```python
from build123d import *

# Parameters (mm, degrees)
BOSS_EXTRU_1_DEPTH           = 80
ENL_V_MAT_EXTRU_1_DEPTH      = 95.994736696
D_GAGEMENT_M11_D             = 16
D_GAGEMENT_M11_DEPTH         = 72
D_GAGEMENT_M11_TIP           = 4.618802154
ENL_V_MAT_EXTRU_2_REACH      = 91.582
ENL_V_MAT_EXTRU_2_END_RADIUS = 8
ESQUISSE3_R                  = 5
ENL_V_MAT_EXTRU_3_REACH      = 92.863
ENL_V_MAT_EXTRU_3_END_RADIUS = 8
ESQUISSE7_R                  = 2


with BuildPart() as part:
    # Esquisse1 → Boss.-Extru.1 (new body)
    with BuildSketch(Plane.XY):
        Polygon((-16, 0), (16, 0), (16, 32), (8, 40), (-8, 40), (-16, 32), align=None)
    extrude(amount=BOSS_EXTRU_1_DEPTH)

    # Esquisse2 → Enlèv. mat.-Extru.1 (cut, through all)
    with BuildSketch(Plane(origin=(16, 0, 0), x_dir=(0, 0, -1), z_dir=(1, 0, 0))):
        with BuildLine():
            Line((-60, -3), (-60, 0))
            ThreePointArc((-60, 0), (-59.121320344, 2.121320344), (-57, 3))
            Line((-57, 3), (-23, 3))
            ThreePointArc((-23, 3), (-20.878679656, 2.121320344), (-20, 0))
            Line((-20, 0), (-20, -3))
            Line((-20, -3), (-60, -3))
        make_face()
    extrude(amount=-ENL_V_MAT_EXTRU_1_DEPTH, mode=Mode.SUBTRACT)

    # Dégagement M11
    with Locations(Plane.XY.offset(80)):
        with Locations((0, 26)):
            Hole(D_GAGEMENT_M11_D / 2, depth=D_GAGEMENT_M11_DEPTH)
            with Locations((0, 0, -(D_GAGEMENT_M11_DEPTH + D_GAGEMENT_M11_TIP / 2))):  # 120° drill point
                Cone(0, D_GAGEMENT_M11_D / 2, D_GAGEMENT_M11_TIP, mode=Mode.SUBTRACT)

    # Enlèv. mat.-Extru.2: up to this cylinder (the profile starts outside it)
    enl_v_mat_extru_2_end = Plane(origin=(0, 26, 40), z_dir=(0, 0, 1)) * Cylinder(ENL_V_MAT_EXTRU_2_END_RADIUS, 200.164, mode=Mode.PRIVATE)
    # Esquisse3 → Enlèv. mat.-Extru.2 (cut, up to the surface)
    with BuildSketch(Plane.XZ.offset(-3), mode=Mode.PRIVATE) as enl_v_mat_extru_2_sk1:
        with Locations(Location((0, 40, 0), (0, 0, 270))):
            Circle(ESQUISSE3_R)
    enl_v_mat_extru_2_tool1 = extrude(enl_v_mat_extru_2_sk1.sketch, amount=-ENL_V_MAT_EXTRU_2_REACH, mode=Mode.PRIVATE) - enl_v_mat_extru_2_end
    add(enl_v_mat_extru_2_tool1.solids().sort_by_distance((0, 3, 40))[0], mode=Mode.SUBTRACT)

    # Enlèv. mat.-Extru.3: up to this cylinder (the profile starts outside it)
    enl_v_mat_extru_3_end = Plane(origin=(0, 26, 10), z_dir=(0, 0, 1)) * Cylinder(ENL_V_MAT_EXTRU_3_END_RADIUS, 202.726, mode=Mode.PRIVATE)
    # Esquisse7 → Enlèv. mat.-Extru.3 (cut, up to the surface)
    with BuildSketch(Plane.XZ, mode=Mode.PRIVATE) as enl_v_mat_extru_3_sk1:
        with Locations(Location((0, 10, 0), (0, 0, 270))):
            Circle(ESQUISSE7_R)
    enl_v_mat_extru_3_tool1 = extrude(enl_v_mat_extru_3_sk1.sketch, amount=-ENL_V_MAT_EXTRU_3_REACH, mode=Mode.PRIVATE) - enl_v_mat_extru_3_end
    add(enl_v_mat_extru_3_tool1.solids().sort_by_distance((0, 0, 10))[0], mode=Mode.SUBTRACT)


solid = part.part
```
Check sheet for the modelled part. Datum: model origin and axes. Units: mm. A direction names the side the tool comes from. Coordinates: 2 decimals unless noted, no trailing zeros. Order: outer loops, then holes, each group sorted by start corner. A loop starts at its lowest first (then second) coordinate and runs counter-clockwise, first axis right, second up. Notation, with made-up numbers: M -8,41 L 31,41 A27 ccw 31,64 Z; hole C 14.25,11 d11. An arc over 180 degrees is marked long. One line per question, with ' | ' between items. Start each with the question number.
Item 1: Sectioned sample at D-D on z = 10. Record the cut outline in (x, y), and give its area (3 significant figures).
Item 2: Gauge pin test, flat ends, axial feed: P1, Ø10, axis at x = -0.5, z = 39, coming from the -Y side; P2, Ø5, axis at x = 1.5, z = 41, coming from the -Y side; P3, Ø6, axis at x = 0, z = 40, coming from the -Y side. Record the tip position at first contact, or that the pin passes through.
Item 3: Mould release check, pull along Y, two halves, no side actions. Record for faces 4 (the flat face through (0, 16, 80)), 5 (the conical face through (-0.2, 27.4, 4.2)), 6 (the cylindrical face through (0.22, 2.14, 20.9)): pulls with the +Y half, pulls with the -Y half, needs draft (parallel to the pull), parting line crosses it, or undercut.
Item 4: Sectioned sample at B-B on x = -11. Record the cut outline in (y, z), and give its area (3 significant figures).
Item 5: Sectioned sample at C-C on y = 5. Record the cut outline in (x, z), and give its area (3 significant figures).
Item 6: Access from +Z, -Z, +X, -X, +Y, -Y to the whole of each face (thin tool, end or side, straight path). Record for faces 1 (the flat face through (4, 3, 44)), 2 (the cylindrical face through (1.041, 33.932, 43.496)), 3 (the cylindrical face through (-1.2, 9, 11.6)).
Item 7: Material ranges on line 1 (Z direction, x = 0, y = 14); line 2 (X direction, y = 2, z = 10); line 3 (X direction, y = 11.25, z = 40), recorded low to high.
Item 8: Sectioned sample at A-A on z = 47. Record the cut outline in (x, y), and give its area (3 significant figures).
Answer below:
1) outline: M -16,0 L -2,0 L -2,18.25 A8 cw long 2,18.25 L 2,0 L 16,0 L 16,32 L 8,40 L -8,40 L -16,32 Z | area: 943 mm^2
2) P1: stops at y = 3 | P2: stops at y = 32.93 | P3: stops at y = 33.42
3) face 4: needs draft | face 5: undercut | face 6: pulls with the -Y half
4) outline: M 0,0 L 37,0 L 37,80 L 0,80 L 0,60 A3 cw 3,57 L 3,23 A3 cw 0,20 Z | area: 2,840 mm^2
5) outline: M -16,0 L 16,0 L 16,80 L -16,80 Z; hole C 0,40 d10; hole C 0,10 d4 | area: 2,470 mm^2
6) face 1: +X, -X, -Y | face 2: +Z | face 3: -Y
7) line 1: z = 0 to 8, 12 to 35, 45 to 80 | line 2: x = -16 to -2, 2 to 16 | line 3: x = -16 to -5, 5 to 16
8) outline: M -16,3 L 16,3 L 16,32 L 8,40 L -8,40 L -16,32 Z; hole C 0,26 d16 | area: 919 mm^2
